Geometry check sheet. Reference: drawing and pictorial views, mm from the part's lowest x, y, z. A direction names the side the tool comes from. Round coordinates to 2 decimals unless told otherwise and drop trailing zeros. Order: outer loops, then holes, each group sorted by start corner. A loop starts at its lowest first (then second) coordinate and runs counter-clockwise, first axis right, second up.
(1) Sectioned sample at C-C, the plane x = 24. Enter the section's corners in (y, z).
(2) Thickness scan on probe 1 along Y at (x, z) = (24, 2.2); probe 2 along Z at (x, y) = (2.5, 11.5); probe 3 along Y at (x, z) = (27.5, 12). Record the ranges inside material, lowest first.
(3) Sectioned sample at B-B, the plane y = 15. Enter the section's corners in (x, z), and give its area (3 significant figures).
(4) Tool access check on the marked faces 3 and 4. Record the directions out of +Z, -Z, +X, -X, +Y, -Y that give a thin tool (end or side, any length) a straight path to the whole face; none if there is none.
(5) Depth check by flat-ended pin: pin 1 (4 mm diameter, centred on x = 24, y = 15, fed in from -Z); pin 2 (12 mm diameter, centred on x = 20, y = 7.5, fed in from +Z); pin 3 (3 mm diameter, centred on x = 19.5, z = 16, fed in from -Y). Enter the tip coordinate at first touch or a pass-through.
(6) Sectioned sample at A-A, the plane x = 6. Enter the section's corners in (y, z), and give its area (3 significant figures).
(7) Sectioned sample at D-D, the plane z = 11. Enter the section's corners in (x, y).
(8) Mould release check, pull along X, two halves, no side actions. Record for the marked faces 1 and 2: released by +X, released by -X, zero draft, split by the parting line, or undercut.
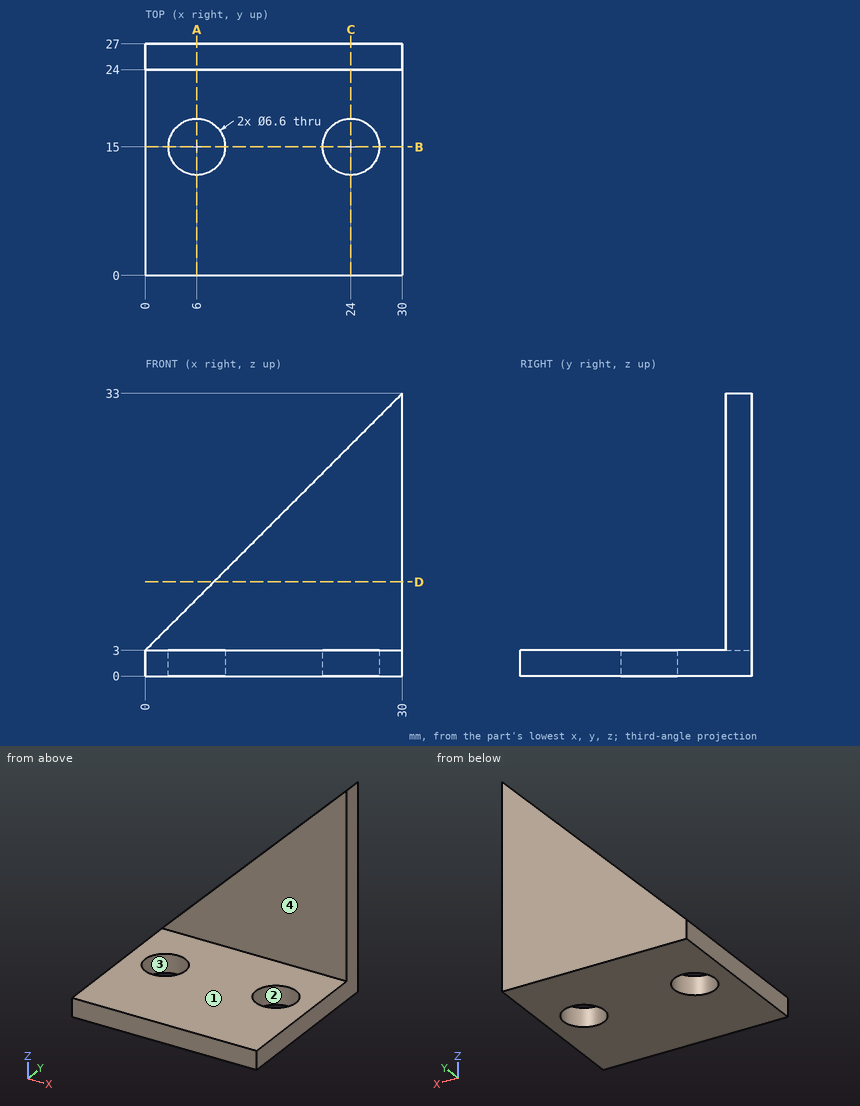
Derived:
1. outline: (0, 0) - (11.7, 0) - (11.7, 3) - (0, 3) - close; (18.3, 0) - (27, 0) - (27, 27) - (24, 27) - (24, 3) - (18.3, 3) - close
2. probe 1: y = 0 to 11.7, 18.3 to 27
2. probe 2: z = 0 to 3
2. probe 3: y = 24 to 27
3. outline: (0, 0) - (2.7, 0) - (2.7, 3) - (0, 3) - close; (9.3, 0) - (20.7, 0) - (20.7, 3) - (9.3, 3) - close; (27.3, 0) - (30, 0) - (30, 3) - (27.3, 3) - close
3. area: 50.4 mm2
4. face 3: +Z, -Z
4. face 4: +Z, +X, -X, -Y
5. pin 1: passes through
5. pin 2: stops at z = 3
5. pin 3: stops at y = 24
6. outline: (0, 0) - (11.7, 0) - (11.7, 3) - (0, 3) - close; (18.3, 0) - (27, 0) - (27, 9) - (24, 9) - (24, 3) - (18.3, 3) - close
6. area: 79.2 mm2
7. outline: (8, 24) - (30, 24) - (30, 27) - (8, 27) - close
8. face 1: zero draft
8. face 2: undercut
